Build history of the part. All positions in model axes, mm. A direction names the side the tool comes from. Round coordinates to 2 decimals unless told otherwise and drop trailing zeros. Order: outer loops, then holes, each group sorted by start corner. A loop starts at its lowest first (then second) coordinate and runs counter-clockwise, first axis right, second up. Notation, with made-up numbers: (-10.5, -21) -> (48.5, -21) arc R19 ccw to (48.5, -15) -> close; hole circle Ø10 at (68.25, 84). An arc over 180 degrees is marked (long way). Use a Markdown table: item, result. Add a question column.
Item 1: Slice it at D-D, the plane y = 3. State how many separate pieces and enclosed holes the cut face has, plus the area to 3 significant figures.
Item 2: 3-axis set-ups, long thin cutter, end or side, ignore diameter. For faces 1 (the face through (4, -12.5, 1)), 2 (the face through (4, -4.5, 0)): which of +Z, -Z, +X, -X, +Y, -Y reach the whole face in a straight line?
Item 3: Probe L1, parallel to Y at x = 3.25, z = -55; L2, parallel to Y at x = 4.75, z = -4; L3, parallel to Z at x = 4, y = 4.25. List the from-to ranges inside material, lowest first.
Item 4: Slice it at A-A, the plane z = 13. Give the cut face in (x, y).
Item 5: Two-plate mould, pull along Z, no slides. Class faces 3 (the face through (8, -5, 1)), 4 (the face through (4, 4.5, 0)), 5 (the face through (3.972, 0.275, -67.497)): released by +Z, released by -Z, zero draft, split by the parting line, or undercut.
Item 6: Slice it at B-B, the plane x = 4.25. Give the cut face in (y, z).
Item 7: Slice it at C-C, the plane z = -47.5. Give the cut face in (x, y).
Item 8: Pin check, flat tips, straight feed: pin 1 (2 mm diameter, centred on x = 3.5, y = -8, fed in from -Z); pin 2 (3 mm diameter, centred on x = 6, y = -9, fed in from +Z). Stop position of each tip, or through.
Autodesk Inventor part; units mm, degrees
ref_plane "YZ Plane" through (0, 0, 0) normal (1, 0, 0) x (0, 1, 0)
ref_plane "XZ Plane" through (0, 0, 0) normal (0, 1, 0) x (-1, 0, 0)
ref_plane "XY Plane" through (0, 0, 0) normal (0, 0, 1) x (1, 0, 0)
sketch "Sketch1" plane through (0, 0, 0) normal (1, 0, 0) x (0, 1, 0)
  line L0 (12.5, 55) -> (-12.5, 55)
  line L1 (-12.5, 55) -> (-12.5, -55)
  line L2 (-12.5, -55) -> (12.5, -55)
  line L3 (12.5, -55) -> (12.5, 55)
  arc A0 (12.5, 55) -> (-12.5, 55) centre (0, 55) ccw
  arc A1 (-12.5, -55) -> (12.5, -55) centre (0, -55) ccw
  line L4 (4, 55) -> (-4, 55)
  circle A2 centre (0, 55) radius 5.25
  circle A3 centre (0, -55) radius 5.25
  line L5 (4.5, 25) -> (-4.5, 25)
  line L6 (-4.5, 25) -> (-4.5, -25)
  line L7 (-4.5, -25) -> (4.5, -25)
  line L8 (4.5, -25) -> (4.5, 25)
  line L9 (4.5, 25) -> (-4.5, -25) construction
  line L10 (-4.5, 25) -> (4.5, -25) construction
  arc A4 (4.5, -25) -> (-4.5, -25) centre (0, -33.9303) ccw
  arc A5 (-4.5, 25) -> (4.5, 25) centre (0, 33.9303) ccw
  point P0 (0, 0)
  point P1 (12.5, 0)
  dimension "d0" = 110
  dimension "d1" = 55
  dimension "d2" = 12.5
  dimension "d3" = 25
  dimension "d27" = 12.5
  dimension "d28" = 10.5
  dimension "d29" = 10.5
  dimension "d31" = 55
  dimension "d40" = 50
  dimension "d42" = 8
  dimension "d43" = 10
  dimension "d44" = 10
extrude "Extrusion1" add sketch "Sketch1" along normal blind 8 contours L3 L2 A3 L1 L0 A2 | L0 A2 A0 | A1 L2 A3 | A5 L5 | L7 A4
fillet "Fillet3" radius 2 8 edges at (8, 0, 67.5) (8, -12.5, 0) (8, 0, -67.5) (8, 12.5, 0) (0, 0, 67.5) (0, -12.5, 0) (0, 0, -67.5) (0, 12.5, 0)
equation "\"d0\" = FEMUR_LENGTH"
equation "\"d3\" = FEMUR_WIDTH"
equation "\"d17\" = FEMUR_HEIGHT"
equation "\"d25\" = PART_FILLET"
properties part number "FemurHornSide"
Check sheet entries:
| question | item | result |
|---|---|---|
| 1 | separate pieces | 4 |
| 1 | enclosed holes | 0 |
| 1 | area | 542 mm2 |
| 2 | face 1 | +Z, -Z, +X, -X, -Y |
| 2 | face 2 | +X, -X |
| 3 | L1 | -12.5 to -5.25, 5.25 to 12.5 |
| 3 | L2 | -12.5 to -4.5, 4.5 to 12.5 |
| 3 | L3 | -66.76 to -58.08, -51.92 to -24.88, 24.88 to 51.92, 58.08 to 66.76 |
| 4 | outline | (0, -10.5) arc R2 ccw to (2, -12.5) -> (6, -12.5) arc R2 ccw to (8, -10.5) -> (8, -4.5) -> (0, -4.5) -> close; (0, 4.5) -> (8, 4.5) -> (8, 10.5) arc R2 ccw to (6, 12.5) -> (2, 12.5) arc R2 ccw to (0, 10.5) -> close |
| 5 | face 3 | zero draft |
| 5 | face 4 | undercut |
| 5 | face 5 | released by -Z |
| 6 | outline | (-12.5, -55) arc R12.5 ccw to (12.5, -55) -> (12.5, 55) arc R12.5 ccw to (-12.5, 55) -> close; hole circle Ø10.5 at (0, -55); hole circle Ø10.5 at (0, 55); hole (-4.5, -25) arc R10 cw to (4.5, -25) -> (4.5, 25) arc R10 cw to (-4.5, 25) -> close |
| 7 | outline | (0, -10.5) arc R2 ccw to (2, -12.5) -> (6, -12.5) arc R2 ccw to (8, -10.5) -> (8, 10.5) arc R2 ccw to (6, 12.5) -> (2, 12.5) arc R2 ccw to (0, 10.5) -> close |
| 8 | pin 1 | z = -65.36 |
| 8 | pin 2 | z = 65 |
